Geometry: final body of the model. Coordinates: model frame, mm. Coordinates: 2 decimals unless noted, no trailing zeros. Write each loop counter-clockwise with the first axis right and the second up, starting at its lowest first coordinate (ties: lowest second). Pieces come first, ordered by that corner, then holes.
from build123d import *

# Parameters (mm, degrees)
PAD025_DEPTH    = 3
SKETCH041_R     = 5.4
POCKET015_DEPTH = 5
SKETCH042_W     = 6
SKETCH042_H     = 4
POCKET016_DEPTH = 5


with BuildPart() as part:
    # Sketch040 (on Face5 of Binder007) → Pad025 (new body)
    with BuildSketch(Plane.XY.offset(3)):
        Polygon((12, 52), (-12, 52), (-15, 49), (-15, 42), (-39, 42), (-42, 39), (-42, -39), (-39, -42), (-15, -42), (-15, -49), (-12, -52), (12, -52), (15, -49), (15, -42), (39, -42), (42, -39), (42, 39), (39, 42), (15, 42), (15, 49), align=None)
    extrude(amount=PAD025_DEPTH)

    # Sketch041 (on Face22 of Pad025) → Pocket015 (cut)
    with BuildSketch(Plane.XY.offset(6)):
        with Locations((-30, 30)):
            Circle(SKETCH041_R)
        with Locations((-10, 30)):
            Circle(SKETCH041_R)
        with Locations((10, 30)):
            Circle(SKETCH041_R)
        with Locations((30, 30)):
            Circle(SKETCH041_R)
        with Locations((-30, 10)):
            Circle(SKETCH041_R)
        with Locations((-10, 10)):
            Circle(SKETCH041_R)
        with Locations((10, 10)):
            Circle(SKETCH041_R)
        with Locations((30, 10)):
            Circle(SKETCH041_R)
        with Locations((-30, -10)):
            Circle(SKETCH041_R)
        with Locations((-10, -10)):
            Circle(SKETCH041_R)
        with Locations((10, -10)):
            Circle(SKETCH041_R)
        with Locations((30, -10)):
            Circle(SKETCH041_R)
        with Locations((-30, -30)):
            Circle(SKETCH041_R)
        with Locations((-10, -30)):
            Circle(SKETCH041_R)
        with Locations((10, -30)):
            Circle(SKETCH041_R)
        with Locations((30, -30)):
            Circle(SKETCH041_R)
    extrude(amount=-POCKET015_DEPTH, mode=Mode.SUBTRACT)

    # Sketch042 (on Face5 of Pocket015) → Pocket016 (cut)
    with BuildSketch(Plane.XY.offset(6)):
        with Locations((-7, -47)):
            Rectangle(SKETCH042_W, SKETCH042_H)
        with Locations((7, -47)):
            Rectangle(SKETCH042_W, SKETCH042_H)
        with Locations((-7, 47)):
            Rectangle(SKETCH042_W, SKETCH042_H)
        with Locations((7, 47)):
            Rectangle(SKETCH042_W, SKETCH042_H)
    extrude(amount=-POCKET016_DEPTH, mode=Mode.SUBTRACT)


solid = part.part
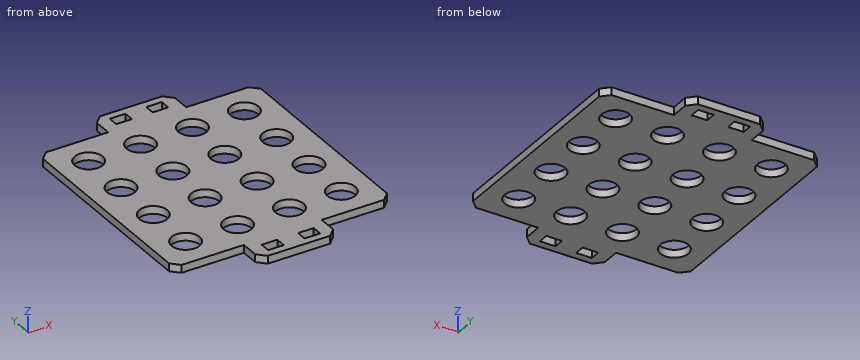
Item 1: Pin query (flat end, axial travel): pin 1 (0.9 mm diameter, centred on y = 46.5, z = 4, fed in from +X); pin 2 (0.9 mm diameter, centred on x = -21.5, z = 4, fed in from -Y); pin 3 (6.5 mm diameter, centred on x = -10, y = -30, fed in from -Z); pin 4 (1.5 mm diameter, centred on y = 46.5, z = 4, fed in from -X). Return the tip coordinate at first contact, or that it passes through.
Derived:
pin 1: stops at x = 15
pin 2: stops at y = -42
pin 3: passes through
pin 4: stops at x = -15
Item 2: Material intervals for probe 1 along Y at (x, z) = (30.5, 5.1); probe 2 along X at (y, z) = (25.5, 3.65); probe 3 along X at (y, z) = (-31, 3.7), sorted ascending.
Derived:
probe 1: y = -42 to -35.38, -24.62 to -15.38, -4.62 to 4.62, 15.38 to 24.62, 35.38 to 42
probe 2: x = -42 to -32.98, -27.02 to -12.98, -7.02 to 7.02, 12.98 to 27.02, 32.98 to 42
probe 3: x = -42 to -35.31, -24.69 to -15.31, -4.69 to 4.69, 15.31 to 24.69, 35.31 to 42
Item 3: Section C-C, the plane z = 5. State how many separate pieces and enclosed holes the cut face has, plus the area to 3 significant figures.
Derived:
separate pieces: 1
enclosed holes: 20
area: 6,060 mm2
Item 4: Section A-A, the plane x = 30. Output: boundary loops of the cut face in (y, z), plus the area to 3 significant figures.
Derived:
outline: (-42, 3) - (-35.4, 3) - (-35.4, 6) - (-42, 6) - close; (-24.6, 3) - (-15.4, 3) - (-15.4, 6) - (-24.6, 6) - close; (-4.6, 3) - (4.6, 3) - (4.6, 6) - (-4.6, 6) - close; (15.4, 3) - (24.6, 3) - (24.6, 6) - (15.4, 6) - close; (35.4, 3) - (42, 3) - (42, 6) - (35.4, 6) - close
area: 122 mm2
